from build123d import *

# Parameters (mm, degrees)
SKETCH2_W           = 206.36
SKETCH2_H           = 173.64
BOSS_EXTRUDE1_DEPTH = 3.18
CUT_EXTRUDE1_DEPTH  = 135.884903529
SKETCH9_W           = 10
SKETCH9_H           = 3.18
BOSS_EXTRUDE4_DEPTH = 3.18
SKETCH11_R          = 1.47
CUT_EXTRUDE3_DEPTH  = 137.953367246


with BuildPart() as part:
    # Sketch2 → Boss-Extrude1 (new body)
    with BuildSketch(Plane.XY):
        Rectangle(SKETCH2_W, SKETCH2_H)
    extrude(amount=BOSS_EXTRUDE1_DEPTH)

    # Sketch3 → Cut-Extrude1 (cut, through all)
    with BuildSketch(Plane.XY.offset(3.18)):
        Polygon((-95.32, -1.47), (-95.32, -3.25), (-97.92, -3.25), (-97.92, -1.47), (-100, -1.47), (-100, -5), (-103.18, -5), (-103.18, 5), (-100, 5), (-100, 1.47), (-97.92, 1.47), (-97.92, 3.25), (-95.32, 3.25), (-95.32, 1.47), (-93.25, 1.47), (-93.25, -1.47), align=None)
    cut_extrude1 = extrude(amount=-CUT_EXTRUDE1_DEPTH, mode=Mode.SUBTRACT)

    # Sketch9 → Boss-Extrude4 (add)
    with BuildSketch(Plane(origin=(0, 86.82, 0), x_dir=(1, 0, 0), z_dir=(0, 1, 0))):
        with Locations((0, -1.59)):
            Rectangle(SKETCH9_W, SKETCH9_H)
    boss_extrude4 = extrude(amount=BOSS_EXTRUDE4_DEPTH)

    # Sketch11 → Cut-Extrude3 (cut, through all)
    with BuildSketch(Plane.XY.offset(3.18)):
        with Locations((0, 88.25)):
            Circle(SKETCH11_R)
    cut_extrude3 = extrude(amount=-CUT_EXTRUDE3_DEPTH, mode=Mode.SUBTRACT)

    # Mirror1: Cut-Extrude1 across plane
    add(cut_extrude1.mirror(Plane(origin=(0, 0, 0), x_dir=(0, 0, 1), z_dir=(1, 0, 0))), mode=Mode.SUBTRACT)

    # Mirror2: Boss-Extrude4, Cut-Extrude3 across plane
    add(boss_extrude4.mirror(Plane.ZX))
    add(cut_extrude3.mirror(Plane.ZX), mode=Mode.SUBTRACT)


solid = part.part
Geometry check sheet. Reference: the model listing, model coordinates, mm. Give positions to 0.01 mm unless a question says otherwise; leave off trailing zeros. Loops run counter-clockwise (first coordinate to the right, second up) from the corner with the lowest first, then second, coordinate; pieces in that order, holes last. Notation, with made-up numbers: M 50.5,85 L 90.5,85 A9 ccw 90.5,101 Z; hole C -13,88.5 d6. An arc over 180 degrees is marked long. Answer as a JSON object with one key per item and string values. Group by question number.
Item 1: Gauge pin test, flat ends, axial feed: pin 1 (1.7 mm diameter, centred on x = -94.5, z = 2, fed in from -Y); pin 2 (1 mm diameter, centred on x = 98.5, z = 1.5, fed in from +Y); pin 3 (1.4 mm diameter, centred on y = -2.5, z = 2, fed in from -X). Record the tip position at first contact, or that the pin passes through.
Item 2: Material ranges on L1, parallel to Y at x = 0, z = 2; L2, parallel to X at y = -88.25, z = 1.35; L3, parallel to Y at x = 95.5, z = 0.6, recorded low to high.
Item 3: Sectioned sample at B-B on x = 66. Record the boundary of the cut face in (y, z).
Item 4: Sectioned sample at A-A on z = 2.05. Give the number of separate pieces and of enclosed holes in the cut face, plus the area to 3 significant figures.
Findings below:
{
 "1": {"pin 1": "y = -86.82", "pin 2": "y = 86.82", "pin 3": "x = -100"},
 "2": {"L1": "-90 to -89.72, -86.78 to 86.78, 89.72 to 90", "L2": "-5 to -1.47, 1.47 to 5", "L3": "-86.82 to -3.25, 3.25 to 86.82"},
 "3": {"outline": "M -86.82,0 L 86.82,0 L 86.82,3.18 L -86.82,3.18 Z"},
 "4": {"separate pieces": "1", "enclosed holes": "2", "area": "35,800 mm2"}
}
